Job drawing, mm, ordinate dimensions from the low corner. One solid piece. Give positions to 0.01 mm unless a question says otherwise; leave off trailing zeros. Write each loop counter-clockwise with the first axis right and the second up, starting at its lowest first coordinate (ties: lowest second). Pieces come first, ordered by that corner, then holes. Notation, with made-up numbers: M -4,44 L 20,44 A25 cw 20,56 Z; hole C 82.5,-36.5 d4. An arc over 180 degrees is marked long. Use CSV: the item, a comma, the result in double quotes. Start each with the question number.
Item 1: Pin check, flat tips, straight feed: pin 1 (0.8 mm diameter, centred on y = 12.5, z = 0.5, fed in from -X); pin 2 (1.5 mm diameter, centred on x = 104, y = 5.5, fed in from -Z). Stop position of each tip, or through.
Item 2: Cut at A-A (y = 5.5). List the corners of the cut face in (x, z), then the cut area to 3 significant figures.
Item 3: Drill centre line: line 1 (X direction, y = 17.5, z = 0.7). Where is it in solid material? Low to high. Write a range as [from, to].
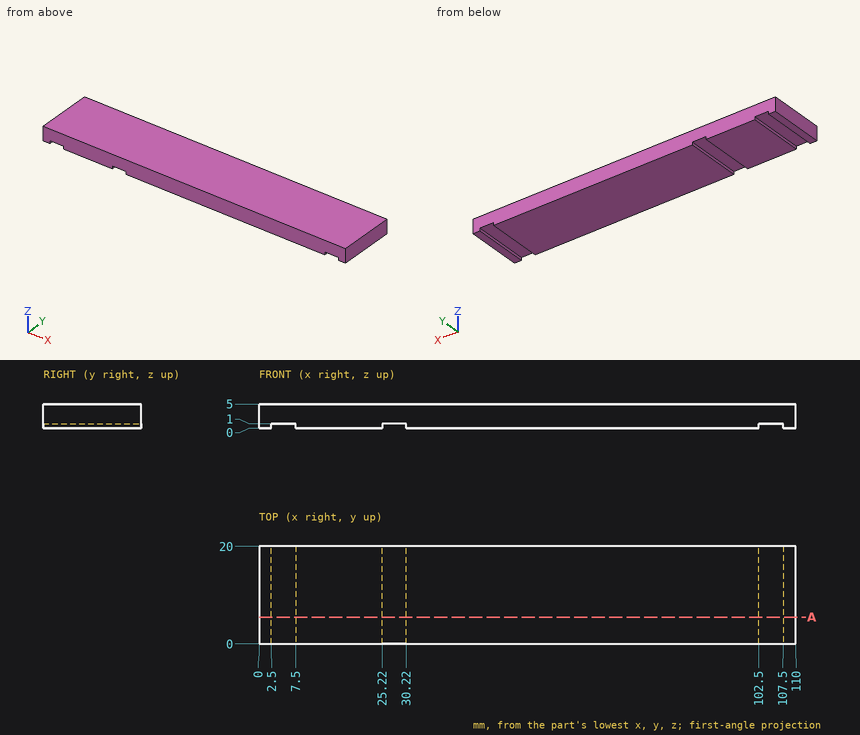
Worked answers:
1,pin 1,"stops at x = 0"
1,pin 2,"stops at z = 1"
2,outline,"M 0,0 L 2.5,0 L 2.5,1 L 7.5,1 L 7.5,0 L 25.22,0 L 25.22,1 L 30.22,1 L 30.22,0 L 102.5,0 L 102.5,1 L 107.5,1 L 107.5,0 L 110,0 L 110,5 L 0,5 Z"
2,area,"535 mm^2"
3,line 1,"x = [0, 2.5], [7.5, 25.22], [30.22, 102.5], [107.5, 110]"
